Source: CAD feature listing. Evaluate the final solid. Frame: model axes, mm. Face numbers are marked on the shaded views. A direction names the side the tool comes from. Give positions to 0.01 mm unless a question says otherwise; leave off trailing zeros. Loops run counter-clockwise (first coordinate to the right, second up) from the corner with the lowest first, then second, coordinate; pieces in that order, holes last. Notation, with made-up numbers: M 64,32 L 82,32 A24 cw 82,51 Z; hole C 49.5,73.25 d2. An arc over 180 degrees is marked long. Put each result on its own line as item: value. Start each with the question number.
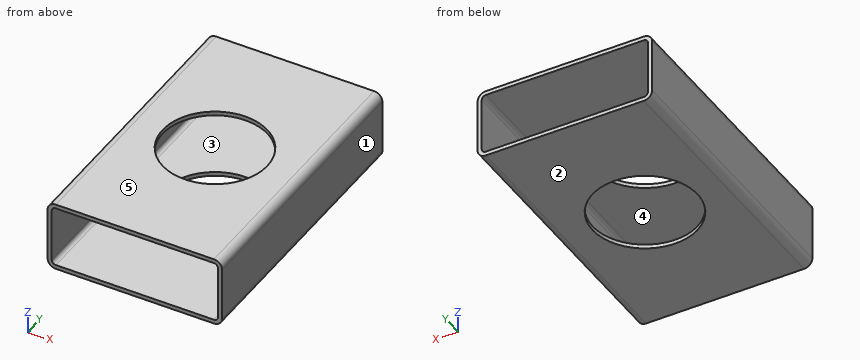
```python
from build123d import *

# Parameters (mm, degrees)
F1_DEPTH = 203.2
F2_R     = 38.1
F3_DEPTH = 50.801


with BuildPart() as f1:
    # F0 (on Front) → F1 (new body)
    with BuildSketch(Plane.XZ):
        with BuildLine():
            Line((-57.5, -25.4), (57.5, -25.4))
            ThreePointArc((57.5, -25.4), (61.742641, -23.642641), (63.5, -19.4))
            Line((63.5, -19.4), (63.5, 19.4))
            ThreePointArc((63.5, 19.4), (61.742641, 23.642641), (57.5, 25.4))
            Line((57.5, 25.4), (-57.5, 25.4))
            ThreePointArc((-57.5, 25.4), (-61.742641, 23.642641), (-63.5, 19.4))
            Line((-63.5, 19.4), (-63.5, -19.4))
            ThreePointArc((-63.5, -19.4), (-61.742641, -23.642641), (-57.5, -25.4))
        make_face()
        with BuildLine():
            ThreePointArc((60.5, -19.4), (59.62132, -21.52132), (57.5, -22.4))
            Line((57.5, -22.4), (-57.5, -22.4))
            ThreePointArc((-57.5, -22.4), (-59.62132, -21.52132), (-60.5, -19.4))
            Line((-60.5, -19.4), (-60.5, 19.4))
            ThreePointArc((-60.5, 19.4), (-59.62132, 21.52132), (-57.5, 22.4))
            Line((-57.5, 22.4), (57.5, 22.4))
            ThreePointArc((57.5, 22.4), (59.62132, 21.52132), (60.5, 19.4))
            Line((60.5, 19.4), (60.5, -19.4))
        make_face(mode=Mode.SUBTRACT)
    extrude(amount=F1_DEPTH)

    # F2 (on face) → F3 (cut, through all)
    with BuildSketch(Plane.XY.offset(25.4)):
        with Locations((0, -101.6)):
            Circle(F2_R)
    extrude(amount=-F3_DEPTH, mode=Mode.SUBTRACT)


solid = f1.part
```
1. Section A-A, the plane z = 5.5. Output: boundary loops of the cut face in (x, y).
2. Section D-D, the plane y = -101.6. Output: boundary loops of the cut face in (x, z).
3. Section B-B, the plane x = 47.5. Output: boundary loops of the cut face in (y, z).
4. Ray query, line 1 (Z direction, x = 38, y = -157); line 2 (X direction, y = -142.5, z = -4); line 3 (Y direction, x = 0, z = -23.75). Return the intervals inside material, ascending.
5. Pull-direction query (Z, two-part tool) for the marked faces 1, 2 and 3; classes: released by +Z, released by -Z, zero draft, split by the parting line, or undercut.
6. Section C-C, the plane y = -56. Output: boundary loops of the cut face in (x, z), plus the area to 3 significant figures.
7. Set-up query: the marked faces 4 and 5. Return all of +Z, -Z, +X, -X, +Y, -Y with unobstructed straight access to the full face (end or side cutting, diameter ignored); none if empty.
Results found:
1. outline: M -63.5,-203.2 L -60.5,-203.2 L -60.5,0 L -63.5,0 Z; M 60.5,-203.2 L 63.5,-203.2 L 63.5,0 L 60.5,0 Z
2. outline: M -63.5,-19.4 A6 ccw -57.5,-25.4 L -38.1,-25.4 L -38.1,-22.4 L -57.5,-22.4 A3 cw -60.5,-19.4 L -60.5,19.4 A3 cw -57.5,22.4 L -38.1,22.4 L -38.1,25.4 L -57.5,25.4 A6 ccw -63.5,19.4 Z; M 38.1,-25.4 L 57.5,-25.4 A6 ccw 63.5,-19.4 L 63.5,19.4 A6 ccw 57.5,25.4 L 38.1,25.4 L 38.1,22.4 L 57.5,22.4 A3 cw 60.5,19.4 L 60.5,-19.4 A3 cw 57.5,-22.4 L 38.1,-22.4 Z
3. outline: M -203.2,-25.4 L 0,-25.4 L 0,-22.4 L -203.2,-22.4 Z; M -203.2,22.4 L 0,22.4 L 0,25.4 L -203.2,25.4 Z
4. line 1: -25.4 to -22.4, 22.4 to 25.4
4. line 2: -63.5 to -60.5, 60.5 to 63.5
4. line 3: -203.2 to -139.7, -63.5 to 0
5. face 1: zero draft
5. face 2: released by -Z
5. face 3: undercut
6. outline: M -63.5,-19.4 A6 ccw -57.5,-25.4 L 57.5,-25.4 A6 ccw 63.5,-19.4 L 63.5,19.4 A6 ccw 57.5,25.4 L -57.5,25.4 A6 ccw -63.5,19.4 Z; hole M -60.5,-19.4 A3 ccw -57.5,-22.4 L 57.5,-22.4 A3 ccw 60.5,-19.4 L 60.5,19.4 A3 ccw 57.5,22.4 L -57.5,22.4 A3 ccw -60.5,19.4 Z
6. area: 1,010 mm²
7. face 4: +Y, -Y
7. face 5: +Z, +X, -X, +Y, -Y
